```python
from build123d import *

# Parameters (mm, degrees)
SKETCH1_W                       = 28.58
SKETCH1_H                       = 50
BOSS_EXTRUDE1_DEPTH             = 12.5
SKETCH2_W                       = 9.53
SKETCH2_H                       = 24.225
SKETCH2_W_2                     = 6.35
CUT_EXTRUDE1_DEPTH              = 39.134028111
FILLET1_R                       = 11.53
SKETCH3_R                       = 6.477
CUT_EXTRUDE2_DEPTH              = 40.975822693
BOSS_EXTRUDE2_DEPTH             = 28.58
SKETCH5_W                       = 28.58
SKETCH5_H                       = 25.775
BOSS_EXTRUDE3_DEPTH             = 80
SKETCH6_R                       = 3.81
CUT_EXTRUDE3_DEPTH              = 100.990331533
CUT_EXTRUDE3_DEPTH_BACK         = 100.990331533
BOSS_EXTRUDE4_REACH             = 110.877
BOSS_EXTRUDE4_DIRECTION_2_REACH = 110.877
TROUS_DE_CENTRAGE_5_0MM1_D      = 5
TROUS_DE_CENTRAGE_5_0MM1_DEPTH  = 10
TROUS_DE_CENTRAGE_5_0MM1_TIP    = 1.502151548
BOSS_EXTRU_1_REACH              = 103.987
FILLET2_R                       = 8
FILLET4_R                       = 4


with BuildPart() as part:
    # Sketch1 → Boss-Extrude1 (new, symmetric)
    with BuildSketch(Plane.XY):
        Rectangle(SKETCH1_W, SKETCH1_H)
    extrude(amount=BOSS_EXTRUDE1_DEPTH, both=True)

    # Sketch2 → Cut-Extrude1 (cut, through all)
    with BuildSketch(Plane(origin=(0, 0, 12.5), x_dir=(-1, 0, 0), z_dir=(0, 0, 1))):
        with Locations((-3.175, -12.8875)):
            Rectangle(SKETCH2_W, SKETCH2_H)
        with Locations((11.115, -12.8875)):
            Rectangle(SKETCH2_W_2, SKETCH2_H)
    extrude(amount=-CUT_EXTRUDE1_DEPTH, mode=Mode.SUBTRACT)

    # Fillet1
    fillet1_edges = [part.edges().sort_by_distance(p)[0] for p in [
        (-4.765, 25, -12.5),
        (-4.765, 25, 12.5),
        (11.115, 25, -12.5),
        (11.115, 25, 12.5),
    ]]
    fillet(fillet1_edges, radius=FILLET1_R)

    # Sketch3 → Cut-Extrude2 (cut, through all)
    with BuildSketch(Plane(origin=(14.29, 0, 0), x_dir=(0, 0, -1), z_dir=(1, 0, 0))):
        with Locations(Location((0, 13.47, 0), (0, 0, 270))):
            Circle(SKETCH3_R)
    extrude(amount=-CUT_EXTRUDE2_DEPTH, mode=Mode.SUBTRACT)

    # Sketch4 → Boss-Extrude2 (add)
    with BuildSketch(Plane(origin=(14.29, 0, 0), x_dir=(0, 0, -1), z_dir=(1, 0, 0))):
        Polygon((18.85, -25), (12.5, -18.65), (12.5, -25), align=None)
    extrude(amount=-BOSS_EXTRUDE2_DEPTH)

    # Sketch5 → Boss-Extrude3 (add)
    with BuildSketch(Plane.XY.offset(12.5)):
        with Locations((0, -12.1125)):
            Rectangle(SKETCH5_W, SKETCH5_H)
    extrude(amount=BOSS_EXTRUDE3_DEPTH)

    # Sketch6 → Cut-Extrude3 (cut, two sides)
    with BuildSketch(Plane(origin=(14.29, 0, 0), x_dir=(0, 0, -1), z_dir=(1, 0, 0))) as cut_extrude3_sk:
        with Locations((-82.5, -12.1125)):
            Circle(SKETCH6_R)
        with Locations((-67.5, -12.1125)):
            Circle(SKETCH6_R)
        with Locations((-52.5, -12.1125)):
            Circle(SKETCH6_R)
    extrude(amount=CUT_EXTRUDE3_DEPTH, mode=Mode.SUBTRACT)
    extrude(cut_extrude3_sk.sketch, amount=-CUT_EXTRUDE3_DEPTH_BACK, mode=Mode.SUBTRACT)

    # Boss-Extrude4: up to this face of the body (flat: up to its plane)
    boss_extrude4_end = Plane(part.part.faces().sort_by_distance((0, -12.1125, 92.5))[0])
    # Sketch7 → Boss-Extrude4 (add, up to the picked face)
    with BuildSketch(Plane(origin=(0, 0, -12.5), x_dir=(-1, 0, 0), z_dir=(0, 0, -1)), mode=Mode.PRIVATE) as boss_extrude4_sk1:
        Polygon((-14.29, -25), (-20.64, -25), (-14.29, -18.65), align=None)
    boss_extrude4_tool1 = split(extrude(boss_extrude4_sk1.sketch, amount=-BOSS_EXTRUDE4_REACH, mode=Mode.PRIVATE), bisect_by=boss_extrude4_end, keep=Keep.BOTH, mode=Mode.PRIVATE)
    boss_extrude4 = boss_extrude4_tool1.solids().sort_by(Axis((16.406667, -22.883333, -12.5), (0, 0, 1)))[0]
    add(boss_extrude4)

    # Boss-Extrude4 direction 2: up to this face of the body (flat: up to its plane)
    boss_extrude4_direction_2_end = Plane(part.part.faces().sort_by_distance((0, -21.825, -15.675))[0])
    # Sketch7 → Boss-Extrude4 direction 2 (add, up to the picked face)
    with BuildSketch(Plane(origin=(0, 0, -12.5), x_dir=(-1, 0, 0), z_dir=(0, 0, -1)), mode=Mode.PRIVATE) as boss_extrude4_direction_2_sk1:
        Polygon((-14.29, -25), (-20.64, -25), (-14.29, -18.65), align=None)
    boss_extrude4_direction_2_tool1 = split(extrude(boss_extrude4_direction_2_sk1.sketch, amount=BOSS_EXTRUDE4_DIRECTION_2_REACH, mode=Mode.PRIVATE), bisect_by=boss_extrude4_direction_2_end, keep=Keep.BOTH, mode=Mode.PRIVATE)
    boss_extrude4_direction_2 = boss_extrude4_direction_2_tool1.solids().sort_by(Axis((16.406667, -22.883333, -12.5), (0, 0, -1)))[0]
    add(boss_extrude4_direction_2)

    # Mirror2: Boss-Extrude4, Boss-Extrude4 direction 2 across plane
    add(boss_extrude4.mirror(Plane(origin=(0, 0, 0), x_dir=(0, 0, 1), z_dir=(1, 0, 0))))
    add(boss_extrude4_direction_2.mirror(Plane(origin=(0, 0, 0), x_dir=(0, 0, 1), z_dir=(1, 0, 0))))

    # Trous de centrage Ø5.0mm1
    with Locations(Plane(origin=(0, -25, 0), x_dir=(-1, 0, 0), z_dir=(0, -1, 0))):
        with Locations((-7.5, 0.534345417), (7.5, 0.534345417), (7.5, -14.465654583), (-7.5, -14.465654583), (-7.5, -29.465654583), (7.5, -29.465654583), (7.5, -44.465654583), (-7.5, -44.465654583)):
            Hole(TROUS_DE_CENTRAGE_5_0MM1_D / 2, depth=TROUS_DE_CENTRAGE_5_0MM1_DEPTH)
            with Locations((0, 0, -(TROUS_DE_CENTRAGE_5_0MM1_DEPTH + TROUS_DE_CENTRAGE_5_0MM1_TIP / 2))):  # 118° drill point
                Cone(0, TROUS_DE_CENTRAGE_5_0MM1_D / 2, TROUS_DE_CENTRAGE_5_0MM1_TIP, mode=Mode.SUBTRACT)

    # Boss.-Extru.1: up to this face of the body (flat: up to its plane)
    boss_extru_1_end = Plane(part.part.faces().sort_by_distance((-14.29, -8.709219679, 38.022768873))[0])
    # Esquisse1 → Boss.-Extru.1 (add, up to the picked face)
    with BuildSketch(Plane(origin=(14.29, 0, 0), x_dir=(0, 0, -1), z_dir=(1, 0, 0)), mode=Mode.PRIVATE) as boss_extru_1_sk1:
        Polygon((-37.5, 30.568839815), (-12.5, 0.775), (-92.5, 0.775), align=None)
    boss_extru_1_tool1 = split(extrude(boss_extru_1_sk1.sketch, amount=-BOSS_EXTRU_1_REACH, mode=Mode.PRIVATE), bisect_by=boss_extru_1_end, keep=Keep.BOTH, mode=Mode.PRIVATE)
    add(boss_extru_1_tool1.solids().sort_by(Axis((14.29, 10.70628, 47.5), (-1, 0, 0)))[0])

    # Fillet2
    fillet2_edges = [part.edges().sort_by_distance(p)[0] for p in [
        (14.29, -18.65, 40),
        (-14.29, -18.65, 40),
        (0, -18.65, -12.5),
    ]]
    fillet(fillet2_edges, radius=FILLET2_R)

    # Fillet4
    fillet4_edges = [part.edges().sort_by_distance(p)[0] for p in [
        (18.636572875, -22.996572875, 92.5),
        (-18.636572875, -22.996572875, 92.5),
        (0, 30.568839815, 37.5),
        (14.29, 15.671919907, 65),
        (14.29, 15.671919907, 25),
        (-14.29, 15.671919907, 65),
        (-14.29, 15.671919907, 25),
        (14.29, -7.280645751, 92.5),
        (-14.89896374, -18.39775896, 92.5),
        (14.89896374, -18.39775896, 92.5),
        (-14.29, 0.775, 0),
        (-14.29, -7.280645751, 92.5),
        (0, 0.775, 92.5),
    ]]
    fillet(fillet4_edges, radius=FILLET4_R)


solid = part.part
```
Input: part model. Units: mm. Frame: model coordinates. A direction names the side the tool comes from. Give positions to 0.01 mm unless a question says otherwise; leave off trailing zeros. Write each loop counter-clockwise with the first axis right and the second up, starting at its lowest first coordinate (ties: lowest second). Pieces come first, ordered by that corner, then holes. Notation, with made-up numbers: (19, -7) - (31, -7) arc R10 ccw to (31, 0) - close; hole circle Ø10 at (78.5, -22). An arc over 180 degrees is marked (long way). Write item = value, one per line. Start each with the question number.
1. Mould query, pull axis Z, two halves, no side actions, for faces 1 (the cylindrical face through (-14.9, -18.4, 75.1)), 2 (the cylindrical face through (-7.825, -19.93, 11.987)), 3 (the cylindrical face through (0.1, 0.5, 91.9)). Classes: released by +Z, released by -Z, zero draft, split by the parting line, or undercut.
2. First-contact query: pin 1 Ø3 at (x, z) = (-7.5, 29.47) entering from -Y; pin 2 Ø8 at (x, z) = (-6, 45.5) entering from -Y; pin 3 Ø6 at (y, z) = (-12.11, 52.5) entering from -X; pin 4 Ø2.5 at (x, z) = (-9, -1.5) entering from +Y. Flat tips, straight axial feed; report the tip coordinate or a pass-through.
3. Ray query, L1, parallel to X at y = 22, z = -5; L2, parallel to Z at x = 7, y = -22; L3, parallel to Y at x = 7.5, z = 80. Return the intervals inside material, ascending.
4. Section query A-A, the plane y = -7. Output: boundary loops of the cut face in (x, z).
5. Access query for faces 4 (the cylindrical face through (13.087, -8.376, 91.359)), 5 (the cylindrical face through (8.654, -19.93, 31.684)), 6 (the cylindrical face through (-4.721, 21.533, 9.212)), 7 (the flat face through (-7.94, 10, 6)), 8 (the flat face through (-1.59, 10, 6)). Directions: +Z, -Z, +X, -X, +Y, -Y. A direction counts if a zero-diameter tool reaches every point of the face in a straight line with its end or side. Return the directions, or none.
6. Section query B-B, the plane x = -3.5. Count the separate pieces of the cut face and the enclosed holes in it, then the cut area to 3 significant figures.
Check sheet entries:
q1.face_1 = zero draft
q1.face_2 = undercut
q1.face_3 = released by +Z
q2.pin_1 = -14.4
q2.pin_2 = -25
q2.pin_3 = through
q2.pin_4 = 25
q3.L1 = -7.94 to -1.59, 7.94 to 14.29
q3.L2 = -15.85 to -2.98, 1.92 to 12.02, 16.92 to 27.02, 31.92 to 42.02, 46.92 to 92.5
q3.L3 = -25 to -14.99, -9.24 to 7.55
q4.outline = (-14.29, -12.5) - (14.29, -12.5) - (14.29, 88.5) arc R4 ccw to (10.29, 92.5) - (-10.29, 92.5) arc R4 ccw to (-14.29, 88.5) - close
q5.face_4 = +Z, +X, +Y
q5.face_5 = -Y
q5.face_6 = +X, -X, +Y
q5.face_7 = -Z, -X, +Y
q5.face_8 = -Z, +Y
q6.separate_pieces = 1
q6.enclosed_holes = 4
q6.area = 4,200 mm2
